Autodesk Inventor part; units mm, degrees
ref_plane "YZ Plane" through (0, 0, 0) normal (1, 0, 0) x (0, 1, 0)
ref_plane "XZ Plane" through (0, 0, 0) normal (0, 1, 0) x (-1, 0, 0)
ref_plane "XY Plane" through (0, 0, 0) normal (0, 0, 1) x (1, 0, 0)
sketch "Sketch1" plane through (0, 0, 0) normal (0, 0, 1) x (1, 0, 0)
  circle A0 centre (0, 0) radius 146.05
  arc A1 (168.91, 0) -> (150.7453, -76.2) centre (0, 0) ccw
  line L0 (6.35, -145.9119) -> (6.35, -168.7906)
  circle A2 centre (-157.48, 0) radius 3.175
  line L1 (6.35, -145.9119) -> (6.35, -150.9919)
  line L2 (6.35, -150.9919) -> (-6.35, -150.9919)
  line L3 (-6.35, -150.9919) -> (-6.35, -161.1519)
  line L4 (-6.35, -161.1519) -> (6.35, -161.1519)
  line L5 (6.35, -150.9919) -> (6.35, -161.1519)
  line L6 (6.35, 145.9119) -> (6.35, 168.7906)
  line L7 (0, 0) -> (0, 200.5264) construction
  line L8 (6.35, 145.9119) -> (6.35, 150.9919) construction
  line L9 (6.35, 150.9919) -> (-12.7, 150.9919)
  line L10 (-12.7, 150.9919) -> (-12.7, 161.1519)
  line L11 (-12.7, 161.1519) -> (6.35, 161.1519)
  line L12 (0, -146.05) -> (0, 0) construction
  line L13 (168.91, 0) -> (168.91, -76.2)
  line L14 (168.91, -76.2) -> (150.7453, -76.2)
  line L15 (0, 0) -> (0, -47.2694) construction
  line L16 (0, -47.2694) -> (158.75, -47.2694) construction
  line L17 (158.75, -42.5069) -> (163.83, -42.5069)
  line L18 (163.83, -42.5069) -> (163.83, -52.0319)
  line L19 (163.83, -52.0319) -> (153.67, -52.0319)
  line L20 (153.67, -52.0319) -> (153.67, -42.5069)
  line L21 (153.67, -42.5069) -> (158.75, -42.5069)
  point P0 (0.0447, 168.91)
  point P1 (6.3947, 145.9099)
  dimension "d51" = 292.1
  dimension "d52" = 337.82
  dimension "d58" = 5.08
  dimension "d59" = 12.7
  dimension "d60" = 10.16
  dimension "d72" = 6.35
  dimension "d73" = 5.08
  dimension "d75" = 19.05
  dimension "d76" = 10.16
  dimension "d77" = 6.35
  dimension "d82" = 76.2
  dimension "d86" = 47.2694
  dimension "d87" = 158.75
  dimension "d89" = 4.7625
  dimension "d90" = 5.08
  dimension "d91" = 9.525
  dimension "d92" = 10.16
  dimension "d93" = 4.7625
extrude "Extrusion15" add sketch "Sketch1" along normal blind 6.35 contours A0 L6 A1 L13 L14 L0
properties part number "TopfemaleHoopSection_v2"
Model file for the job. Use its own axes, mm. A direction names the side the tool comes from. Coordinates: 2 decimals unless noted, no trailing zeros. Loops run counter-clockwise (first coordinate to the right, second up) from the corner with the lowest first, then second, coordinate; pieces in that order, holes last. Notation, with made-up numbers: (-25.5, 73) - (28.5, 73) arc R28 cw to (28.5, 100) - close; hole circle Ø4 at (39, -19). An arc over 180 degrees is marked (long way). Write item = value, one per line. Start each with the question number.
Item 1: Saw through at A-A, the plane x = 108.5. List the corners of the cut face in (y, z).
Item 2: 3-axis set-ups, long thin cutter, end or side, ignore diameter. For faces 5 (the face through (168.91, -38, 3)), 6 (the face through (159, -52.032, 3)): which of +Z, -Z, +X, -X, +Y, -Y reach the whole face in a straight line?
Item 3: Saw through at D-D, the plane y = 87. List the corners of the cut face in (x, z), then the cut area to 3 significant figures.
Item 4: Saw through at B-B, the plane z = 5. List the corners of the cut face in (x, y).
Item 5: Drop flat-ended pins along their axis: pin 1 Ø1.5 at (x, z) = (150, 1.5) entering from +Y; pin 2 Ø2 at (y, z) = (16, 1.5) entering from -X; pin 3 Ø1.9 at (x, z) = (159.5, 3.5) entering from -Y; pin 4 Ø5 at (x, y) = (114.5, -129) entering from -Z. Give the stop position or say it passes through.
Item 6: Wall check: probe 1 along Y at (x, z) = (45, 3); probe 2 along X at (y, z) = (-45, 4.5); probe 3 along Y at (x, z) = (24.5, 3.5). Give the ranges that are in metal, low to high. Write a range as [from, to].
Item 7: Saw through at C-C, the plane x = 61. List the corners of the cut face in (y, z).
Item 8: Pull direction Y, two halves, no side cores. Call faces 1 (the face through (160, -76.2, 3)), 2 (the face through (147, -12, 0)), 3 (the face through (159, -42.507, 3)), 4 (the face through (163.83, -47, 3)): +Y half, -Y half, draft (parallel to the pull), parting line (faces both ways), or undercut.
Answers:
q1.outline = (-129.45, 0) - (-97.77, 0) - (-97.77, 6.35) - (-129.45, 6.35) - close; (97.77, 0) - (129.45, 0) - (129.45, 6.35) - (97.77, 6.35) - close
q2.face_5 = +Z, -Z, +X, +Y, -Y
q2.face_6 = +Z, -Z
q3.outline = (117.31, 0) - (144.78, 0) - (144.78, 6.35) - (117.31, 6.35) - close
q3.area = 174 mm2
q4.outline = (6.35, -168.79) arc R168.91 ccw to (150.75, -76.2) - (168.91, -76.2) - (168.91, 0) arc R168.91 ccw to (6.35, 168.79) - (6.35, 145.91) arc R146.05 cw to (6.35, -145.91) - close; hole (153.67, -52.03) - (163.83, -52.03) - (163.83, -42.51) - (153.67, -42.51) - close
q5.pin_1 = 79.09
q5.pin_2 = 145.06
q5.pin_3 = -76.2
q5.pin_4 = through
q6.probe_1 = [-162.81, -138.94], [138.94, 162.81]
q6.probe_2 = [138.94, 153.67], [163.83, 168.91]
q6.probe_3 = [-167.12, -143.98], [143.98, 167.12]
q7.outline = (-157.51, 0) - (-132.7, 0) - (-132.7, 6.35) - (-157.51, 6.35) - close; (132.7, 0) - (157.51, 0) - (157.51, 6.35) - (132.7, 6.35) - close
q8.face_1 = -Y half
q8.face_2 = draft
q8.face_3 = undercut
q8.face_4 = undercut
